Geometry: final body of the model. Coordinates: model frame, mm. A direction names the side the tool comes from. Give positions to 0.01 mm unless a question says otherwise; leave off trailing zeros. Order: outer loops, then holes, each group sorted by start corner. A loop starts at its lowest first (then second) coordinate and runs counter-clockwise, first axis right, second up. Notation, with made-up numbers: (-37, 88.25) -> (16, 88.25) arc R16 cw to (16, 103.25) -> close; hole circle Ø9 at (43.25, -29.75). An arc over 180 degrees is marked (long way). One line per question, with ' | ' between items.
Autodesk Inventor part; units mm, degrees
ref_plane "YZ Plane" through (0, 0, 0) normal (1, 0, 0) x (0, 1, 0)
ref_plane "XZ Plane" through (0, 0, 0) normal (0, 1, 0) x (-1, 0, 0)
ref_plane "XY Plane" through (0, 0, 0) normal (0, 0, 1) x (1, 0, 0)
sketch "Sketch1" plane through (0, 0, 0) normal (0, 0, 1) x (1, 0, 0)
  line L0 (0, 0) -> (230.251, 0)
  line L1 (230.251, 0) -> (230.251, 107.95)
  line L2 (230.251, 107.95) -> (0, 107.95)
  line L3 (0, 107.95) -> (0, 0)
  line L4 (230.251, 107.95) -> (223.901, 107.95) construction
  line L5 (223.901, 107.95) -> (223.901, 101.6) construction
  line L6 (223.901, 101.6) -> (230.251, 101.6) construction
  line L7 (230.251, 101.6) -> (230.251, 107.95) construction
  line L8 (223.901, 101.6) -> (0, 101.6)
  line L9 (0, 101.6) -> (0, 100.076)
  line L10 (0, 100.076) -> (223.901, 100.076)
  line L11 (223.901, 100.076) -> (223.901, 101.6)
  line L12 (230.251, 0) -> (223.901, 0) construction
  line L13 (223.901, 0) -> (223.901, 35.9833) construction
  line L14 (223.901, 35.9833) -> (230.251, 35.9833) construction
  line L15 (230.251, 35.9833) -> (230.251, 0) construction
  circle A0 centre (223.901, 35.9833) radius 2
  circle A1 centre (223.901, 71.9667) radius 2
  line L16 (230.251, 53.975) -> (0, 53.975) construction
  line L17 (223.901, 6.35) -> (0, 6.35)
  line L18 (0, 7.874) -> (223.901, 7.874)
  line L19 (223.901, 7.874) -> (223.901, 6.35)
  dimension "length" = 230.251
  dimension "height" = 107.95
  dimension "d3" = 6.35
  dimension "d4" = 6.35
  dimension "d5" = 223.901
  dimension "d6" = 1.524
  dimension "spacing" = 35.9833
  dimension "d9" = 6.35
  dimension "TopScrewDiameter" = 4
  dimension "d13" = 35.9833
extrude "Generic Shape" add sketch "Sketch1" along normal blind 12.7
sketch "ScrewCapDiameter" plane through (0, 0, 0) normal (0, 0, -1) x (-1, 0, 0)
  circle A0 centre (-223.901, 71.9667) radius 2
  circle A1 centre (-223.901, 71.9667) radius 4
  circle A2 centre (-223.901, 35.9833) radius 2
  circle A3 centre (-223.901, 35.9833) radius 4
  point P0 (0, 0)
  dimension "d106" = 8
  dimension "d107" = 8
extrude "ScrewCapCountersink" cut sketch "ScrewCapDiameter" against normal blind 4
sketch "PcbNotchDimensions" plane through (0, 0, 12.7) normal (0, 0, 1) x (1, 0, 0)
  line L0 (230.251, 107.95) -> (0, 107.95) construction
  line L1 (230.251, 107.95) -> (223.901, 107.95) construction
  line L2 (223.901, 107.95) -> (223.901, 101.6) construction
  line L3 (223.901, 101.6) -> (230.251, 101.6) construction
  line L4 (230.251, 101.6) -> (230.251, 107.95) construction
  line L5 (223.901, 101.6) -> (1.651, 101.6)
  line L6 (1.651, 101.6) -> (1.651, 99.949)
  line L7 (1.651, 99.949) -> (223.901, 99.949)
  line L8 (223.901, 99.949) -> (223.901, 101.6)
  line L9 (230.251, 0) -> (230.251, 107.95) construction
  line L10 (230.251, 53.225) -> (0, 53.225) construction
  line L11 (0, 107.95) -> (0, 0) construction
  line L12 (223.901, 4.85) -> (1.651, 4.85)
  line L13 (1.651, 4.85) -> (1.651, 6.501)
  line L14 (1.651, 6.501) -> (223.901, 6.501)
  line L15 (223.901, 6.501) -> (223.901, 4.85)
  point P0 (230.251, 106.45)
  point P1 (0, 106.45)
  dimension "d21" = 6.35
  dimension "d22" = 6.35
  dimension "d23" = 222.25
  dimension "PcbThickness" = 1.651
extrude "PCB Notch" cut sketch "PcbNotchDimensions" against normal blind 6.35
sketch "UntappedScrewHoleDimensions" plane through (0, 0, 0) normal (-1, 0, 0) x (0, 0, 1)
  line L0 (0, 0) -> (6.35, 0) construction
  line L1 (6.35, 0) -> (6.35, 35.9833) construction
  line L2 (6.35, 35.9833) -> (0, 35.9833) construction
  line L3 (0, 35.9833) -> (0, 0) construction
  circle A0 centre (6.35, 35.9833) radius 2
  line L4 (0, 107.95) -> (6.35, 107.95) construction
  line L5 (6.35, 107.95) -> (6.35, 71.9667) construction
  line L6 (6.35, 71.9667) -> (0, 71.9667) construction
  line L7 (0, 71.9667) -> (0, 107.95) construction
  circle A1 centre (6.35, 71.9667) radius 2
  dimension "d33" = 6.35
  dimension "d34" = 35.9833
  dimension "ScrewDiameterUntapped" = 4
  dimension "d36" = 6.35
  dimension "d37" = 35.9833
  dimension "d38" = 4
extrude "UntappedScrewDepth" cut sketch "UntappedScrewHoleDimensions" against normal blind 12.7
thread "Thread10"
thread "Thread11"
sketch "Sketch18" plane through (0, 0, 0) normal (0, 0, -1) x (-1, 0, 0)
  line L0 (0, 0) -> (-12.7, 0) construction
  line L1 (-12.7, 0) -> (-12.7, 12.7) construction
  line L2 (-12.7, 12.7) -> (0, 12.7) construction
  line L3 (0, 12.7) -> (0, 0) construction
  line L4 (-12.7, 12.7) -> (-217.551, 12.7)
  line L5 (-217.551, 12.7) -> (-217.551, 95.25)
  line L6 (-217.551, 95.25) -> (-12.7, 95.25)
  line L7 (-12.7, 95.25) -> (-12.7, 12.7)
  dimension "bezel" = 12.7
  dimension "d156" = 12.7
  dimension "d157" = 204.851
  dimension "d158" = 82.55
extrude "Extrusion16" cut sketch "Sketch18" against normal blind 12.7
equation "\"d3\" = 0.5 * thickness"
equation "\"d4\" = 0.5 * thickness"
equation "\"d5\" = length - 0.5 * thickness"
equation "\"spacing\" = 0.333333 * height"
equation "\"d9\" = 0.5 * thickness"
equation "\"d13\" = spacing"
equation "\"d25\" = 0.5 * thickness"
equation "\"d33\" = 0.5 * thickness"
equation "\"d34\" = 0.333333 * height"
equation "\"d36\" = 0.5 * thickness"
equation "\"d37\" = 0.333333 * height"
equation "\"d38\" = ScrewDiameterUntapped"
equation "\"LcdThickness\" = 9.9"
properties part number "2020-03-29 CubeBaseSkeleton"
1) Section B-B on z = 10.75. Return loops of the section in (x, y).
Check result:
outline: (0, 0) -> (230.25, 0) -> (230.25, 107.95) -> (0, 107.95) -> close; hole (1.65, 4.85) -> (223.9, 4.85) -> (223.9, 6.5) -> (1.65, 6.5) -> close; hole (1.65, 99.95) -> (223.9, 99.95) -> (223.9, 101.6) -> (1.65, 101.6) -> close; hole (12.7, 12.7) -> (217.55, 12.7) -> (217.55, 95.25) -> (12.7, 95.25) -> close; hole circle Ø4 at (223.9, 35.98); hole circle Ø4 at (223.9, 71.97)
2) Set-up query: faces 1 (the cylindrical face through (6.26, 73.65, 7.43)), 2 (the flat face through (217.551, 53, 6)), 3 (the flat face through (223, 74, 4)), 4 (the flat face through (114, 4.85, 10)), 5 (the flat face through (106, 10, 0)). Return all of +Z, -Z, +X, -X, +Y, -Y with unobstructed straight access to the full face (end or side cutting, diameter ignored); none if empty.
Check result:
face 1: -X | face 2: +Z, -Z | face 3: -Z | face 4: +Z | face 5: -Z, +X, -X, +Y, -Y
3) Contact query for flat-ended pins moving along their axis: pin 1 Ø2.5 at (x, y) = (222, 73.5) entering from -Z; pin 2 Ø0.5 at (x, y) = (58.5, 6) entering from +Z. Output: stop coordinate, or through.
Check result:
pin 1: stops at z = 4 | pin 2: stops at z = 6.35
4) Material intervals for probe 1 along Y at (x, z) = (60, 9.5); probe 2 along Y at (x, z) = (156, 4.25); probe 3 along X at (y, z) = (17, 9), sorted ascending. Write a range as from..to.
Check result:
probe 1: y = 0..4.85, 6.5..12.7, 95.25..99.95, 101.6..107.95 | probe 2: y = 0..12.7, 95.25..107.95 | probe 3: x = 0..12.7, 217.55..230.25
5) Pull-direction query (Y, two-part tool) for faces 6 (the flat face through (0, 55, 6)), 7 (the cylindrical face through (224.77, 32.08, 1.97)), 8 (the flat face through (117, 107.95, 6)); classes: +Y half, -Y half, draft (parallel to the pull), parting line (faces both ways), or undercut.
Check result:
face 6: draft | face 7: undercut | face 8: +Y half
6) Section A-A on x = 115.5. Return loops of the section in (y, z).
Check result:
outline: (0, 0) -> (12.7, 0) -> (12.7, 12.7) -> (6.5, 12.7) -> (6.5, 6.35) -> (4.85, 6.35) -> (4.85, 12.7) -> (0, 12.7) -> close; (95.25, 0) -> (107.95, 0) -> (107.95, 12.7) -> (101.6, 12.7) -> (101.6, 6.35) -> (99.95, 6.35) -> (99.95, 12.7) -> (95.25, 12.7) -> close
